Design review of the part built by this model. Coordinates are the model's own, in mm. A direction names the side the tool comes from. Coordinates: 2 decimals unless noted, no trailing zeros. Loops run counter-clockwise (first coordinate to the right, second up) from the corner with the lowest first, then second, coordinate; pieces in that order, holes last. Notation, with made-up numbers: M 56.25,44 L 94.25,44 A28 ccw 94.25,71 Z; hole C -30.75,-2.5 d11. An arc over 180 degrees is marked long. Answer as CSV lines item,"result". Start each with the question number.
Autodesk Inventor part; units mm, degrees
ref_plane "YZ Plane" through (0, 0, 0) normal (1, 0, 0) x (0, 1, 0)
ref_plane "XZ Plane" through (0, 0, 0) normal (0, 1, 0) x (-1, 0, 0)
ref_plane "XY Plane" through (0, 0, 0) normal (0, 0, 1) x (1, 0, 0)
sketch "Эскиз1" plane through (0, 0, 0) normal (0, 1, 0) x (-1, 0, 0)
  line L0 (0, 0) -> (12, 0)
  line L1 (12, 0) -> (12, -12)
  line L2 (12, -12) -> (0, -12)
  line L3 (0, -12) -> (0, 0)
  dimension "d0" = 12
  dimension "d1" = 12
extrude "Выдавливание1" add sketch "Эскиз1" along normal blind 2
sketch "Эскиз2" plane through (0, 2, 0) normal (0, 1, 0) x (1, 0, 0)
  line L0 (0, 12) -> (-12, 12)
  line L1 (0, 0) -> (0, 12)
  line L2 (-12, 12) -> (0, 12)
  line L3 (0, 12) -> (0, 0)
  line L4 (0, 0) -> (-12, 0)
  line L5 (-12, 0) -> (-12, 12)
  circle A0 centre (-5.5, 5.5) radius 5.5
  circle A1 centre (-5.5, 5.5) radius 3.5
  line L6 (-12, 12) -> (-12, 0)
  line L7 (-12, 11) -> (0, 11)
  line L8 (-11, 12) -> (-11, 0)
  line L9 (-12, 0) -> (0, 0)
  dimension "d5" = 7
  dimension "d19" = 1
  dimension "d20" = 1
  dimension "d21" = 11
extrude "Выдавливание2" add sketch "Эскиз2" along normal blind 6 contours A1
sketch "Эскиз3" plane through (-5.5, 8, -5.5) normal (0, 1, 0) x (1, 0, 0)
  circle A0 centre (0, 0) radius 3.5
  circle A1 centre (0, 0) radius 1.5
  point P0 (5.5, -5.5)
  dimension "d8" = 3
extrude "Выдавливание3" cut sketch "Эскиз3" against normal blind 8 contours A1
sketch "Эскиз5" plane through (-5.5, 8, -5.5) normal (0, 1, 0) x (1, 0, 0)
  circle A0 centre (0, 0) radius 1.5
  circle A1 centre (0, 0) radius 2.25
  line L0 (2.25, 0) -> (1.125, -1.9486)
  line L1 (1.125, -1.9486) -> (-1.125, -1.9486)
  line L2 (-1.125, -1.9486) -> (-2.25, 0)
  line L3 (-2.25, 0) -> (-1.125, 1.9486)
  line L4 (-1.125, 1.9486) -> (1.125, 1.9486)
  line L5 (1.125, 1.9486) -> (2.25, 0)
  point P0 (5.5, -5.5)
  dimension "d14" = 4.5
extrude "Выдавливание5" cut sketch "Эскиз5" against normal blind 4 contours L0 L1 L2 L3 L4 L5
sketch "Эскиз6" plane through (0, 2, 0) normal (0, 1, 0) x (1, 0, 0)
  line L0 (-12, 0) -> (0, 0)
  line L1 (0, 0) -> (0, 12)
  line L2 (0, 12) -> (0, 0)
  line L3 (0, 0) -> (-12, 0)
  circle A0 centre (-5.5, 5.5) radius 3.5
  arc A1 (-12, 0) -> (0, 12) centre (-10.599, 10.599) ccw
  point P0 (0, 9.1981)
  point P1 (-2.7251, 3.3669)
  point P2 (-3.3669, 2.7251)
  point P3 (-9.1981, 0)
extrude "Выдавливание6" cut sketch "Эскиз6" against normal blind 4 contours A1 A0 L1 L0
properties part number "holder"
Item 1: Add section B-B (x = -8). Give the boundary of the cut face in (y, z).
Item 2: Add section C-C (z = -8.75). Give the boundary of the cut face in (x, y), plus the area to 3 significant figures.
Item 3: Add section D-D (x = -5.5). Give the boundary of the cut face in (y, z).
Item 4: Add section A-A (y = 6). Give the boundary of the cut face in (x, z) (3 decimals), plus the area to 3 significant figures.
Item 5: For line 1 along X through (y, z) = (3, -5.5); line 2 along Y through (x, z) = (-5.25, -9.75), list the stretches that pass through material, from the lowest coordinate up. Write a range as from..to.
Item 6: Mouldability with a two-part tool opening along X and no side actions: class faces 3 (the face through (-3.805, 6.028, -4.539)), 4 (the face through (-6, 8, -3)), 5 (the face through (-12, 1, -6)) as released by +X, released by -X, zero draft, split by the parting line, or undercut.
Item 7: For pin 1 (2 mm diameter, centred on y = 6, z = -10.5, fed in from +X) (3 decimals); pin 2 (0.7 mm diameter, centred on x = -5.5, y = 6.5, fed in from -Z); pin 3 (1 mm diameter, centred on x = -7, y = 5, fed in from -Z); pin 4 (1.1 mm diameter, centred on x = -5.5, y = 5.5, fed in from +Z), all flat-tipped, find the tip position at first contact; note any pin that passes through.
Item 8: For faces 1 (the face through (-7.195, 6.028, -6.461)), 2 (the face through (-6.1, 1, -0.9)), list the 3-axis set-ups (+Z, -Z, +X, -X, +Y, -Y) from which the entire face can be reached by the end or side of a thin tool; tool diameter is ignored.
Response:
1,outline,"M 0,-12 L 2,-12 L 2,-7.95 L 8,-7.95 L 8,-3.05 L 2,-3.05 L 2,-0.23 L 0,-0.23 Z"
2,outline,"M -12,0 L -0.07,0 L -0.07,2 L -4.2,2 L -4.2,8 L -6.8,8 L -6.8,2 L -12,2 Z"
2,area,"39.5 mm²"
3,outline,"M 0,-12 L 2,-12 L 2,-9 L 8,-9 L 8,-7.45 L 4,-7.45 L 4,-7 L 0,-7 Z; M 0,-4 L 4,-4 L 4,-3.55 L 8,-3.55 L 8,-2 L 2,-2 L 2,-1.2 L 0,-1.2 Z"
4,outline,"C -5.5,-5.5 d7; hole M -7.75,-5.5 L -6.625,-7.449 L -4.375,-7.449 L -3.25,-5.5 L -4.375,-3.551 L -6.625,-3.551 Z"
4,area,"25.3 mm²"
5,line 1,"-9..-7, -4..-2"
5,line 2,"0..2"
6,face 3,"undercut"
6,face 4,"zero draft"
6,face 5,"released by -X"
7,pin 1,"through"
7,pin 2,"z = -9"
7,pin 3,"z = -8.85"
7,pin 4,"z = -2"
8,face 1,"+Y"
8,face 2,"+Z, +X, +Y, -Y"
